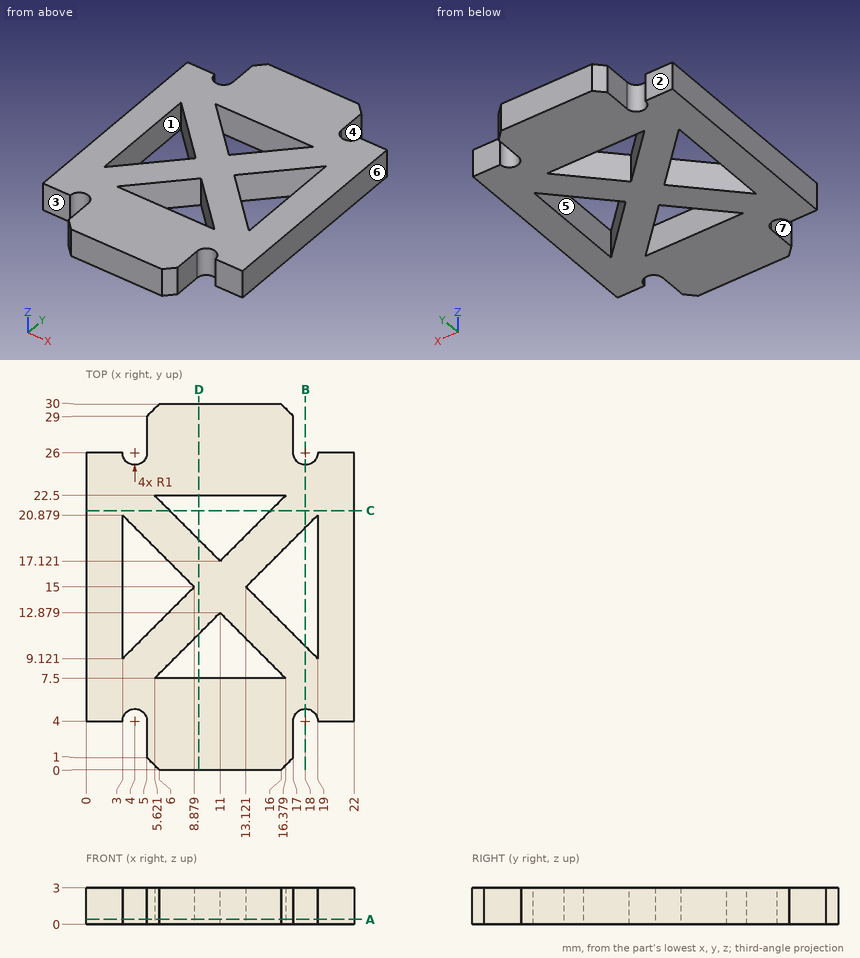
Geometry check sheet. Reference: drawing and pictorial views, mm from the part's lowest x, y, z. A direction names the side the tool comes from. Give positions to 0.01 mm unless a question says otherwise; leave off trailing zeros. Order: outer loops, then holes, each group sorted by start corner. A loop starts at its lowest first (then second) coordinate and runs counter-clockwise, first axis right, second up. Notation, with made-up numbers: M 5.25,-35 L 38.25,-35 A18 ccw 38.25,-9 Z; hole C 50,37.25 d1. An arc over 180 degrees is marked long. Answer in a Markdown table with one row per item.
1) Cross-section at A-A, the plane z = 0.4. Count the separate pieces of the cut face and the enclosed holes in it, plus the area to 3 significant figures.
Filled sheet:
| item | result |
|---|---|
| separate pieces | 1 |
| enclosed holes | 4 |
| area | 445 mm2 |
2) Cross-section at D-D, the plane x = 9.25. Enter the section's corners in (y, z).
Filled sheet:
| item | result |
|---|---|
| outline | M 0,0 L 7.5,0 L 7.5,3 L 0,3 Z; M 11.13,0 L 18.87,0 L 18.87,3 L 11.13,3 Z; M 22.5,0 L 30,0 L 30,3 L 22.5,3 Z |
3) Thickness scan on L1, parallel to X at y = 12.25, z = 1.7; L2, parallel to Y at x = 14, z = 2.1; L3, parallel to Y at x = 14.5, z = 2.85. Record the ranges inside material, lowest first. Write a range as [from, to].
Filled sheet:
| item | result |
|---|---|
| L1 | x = [0, 3], [6.13, 10.37], [11.63, 15.87], [19, 22] |
| L2 | y = [0, 7.5], [9.88, 14.12], [15.88, 20.12], [22.5, 30] |
| L3 | y = [0, 7.5], [9.38, 13.62], [16.38, 20.62], [22.5, 30] |
4) Gauge pin test, flat ends, axial feed: P1, Ø1.5, axis at y = 28, z = 2, coming from the +X side; P2, Ø0.9, axis at x = 20, z = 1.5, coming from the +Y side; P3, Ø1.5, axis at x = 2, z = 2, coming from the -Y side. Record the tip position at first contact, or that the pin passes through.
Filled sheet:
| item | result |
|---|---|
| P1 | stops at x = 17 |
| P2 | stops at y = 26 |
| P3 | stops at y = 4 |
5) Cross-section at B-B, the plane x = 18. Enter the section's corners in (y, z).
Filled sheet:
| item | result |
|---|---|
| outline | M 5,0 L 10.12,0 L 10.12,3 L 5,3 Z; M 19.88,0 L 25,0 L 25,3 L 19.88,3 Z |
6) Access from +Z, -Z, +X, -X, +Y, -Y to the whole of each face (thin tool, end or side, straight path). Record for the marked faces 1, 2, 3 and 4.
Filled sheet:
| item | result |
|---|---|
| face 1 | +Z, -Z |
| face 2 | +Z, -Z, -X, +Y |
| face 3 | +Z, -Z, -X, -Y |
| face 4 | +Z, -Z, +X, +Y |
7) Release check for a two-part mould opening along X. For the marked faces 5, 6 and 7 record: +X half, -X half, draft (parallel to the pull), parting line (faces both ways), or undercut.
Filled sheet:
| item | result |
|---|---|
| face 5 | undercut |
| face 6 | +X half |
| face 7 | -X half |
8) Cross-section at C-C, the plane y = 21.25. Enter the section's corners in (x, z).
Filled sheet:
| item | result |
|---|---|
| outline | M 0,0 L 6.87,0 L 6.87,3 L 0,3 Z; M 15.13,0 L 22,0 L 22,3 L 15.13,3 Z |
